```python
from build123d import *

# Parameters (mm, degrees)
BOSS_EXTRUDE1_DEPTH = 50
SKETCH3_W           = 3.3
SKETCH3_H           = 1
BOSS_EXTRUDE2_DEPTH = 13
BOSS_EXTRUDE3_DEPTH = 53.5
CHAMFER1_START      = -14
CHAMFER1_OUTLINE_W  = 52
CHAMFER1_OUTLINE_H  = 13
CHAMFER1_DEPTH      = 3.182909169
CHAMFER2_SIZE       = 3


with BuildPart() as part:
    # Sketch2 → Boss-Extrude1 (new body)
    with BuildSketch(Plane(origin=(0, 0, 0), x_dir=(1, 0, 0), z_dir=(0, 1, 0))):
        Polygon((-1.7, -2), (-1.7, -15), (-5.7, -15), (-5.7, -2), (-9, -2), (-9, -15), (-13, -15), (-13, 2.680601608), align=None)
    extrude(amount=BOSS_EXTRUDE1_DEPTH)

    # Sketch3 → Boss-Extrude2 (add)
    with BuildSketch(Plane.XY.offset(2)):
        with Locations((-7.35, 0.5)):
            Rectangle(SKETCH3_W, SKETCH3_H)
    extrude(amount=BOSS_EXTRUDE2_DEPTH)

    # Sketch5 → Boss-Extrude3 (add)
    with BuildSketch(Plane.XY.offset(15)):
        Polygon((-13, 0), (-1.7, 0), (-1.7, 14), (-5.7, 14), (-5.7, 1), (-9, 1), (-9, 14), (-13, 14), align=None)
    extrude(amount=BOSS_EXTRUDE3_DEPTH)

    # Mirror1: part across plane


with BuildPart() as part_1:
    add(part.part)
    add(part.part.mirror(Plane(origin=(-0.956063716, 0, 2.308147732), x_dir=(0.9238798691632129, 0, 0.38268261961443256), z_dir=(0.3826826196144326, 0, -0.9238798691632131))))

    # Chamfer1: read off the stored shape, not the designer's step
    # Chamfer1 outline → Chamfer1 (cut)
    with BuildSketch(Plane(origin=(0, 0, 0), x_dir=(0, 1, 0), z_dir=(0.9238798691632129, 0, 0.38268261961443295)).offset(CHAMFER1_START)):
        with Locations((25, 2.5)):
            Rectangle(CHAMFER1_OUTLINE_W, CHAMFER1_OUTLINE_H)
    extrude(amount=CHAMFER1_DEPTH, mode=Mode.SUBTRACT)

    # Chamfer2
    chamfer2_edges = [part_1.edges().sort_by_distance(p)[0] for p in [
        (-13, 32, 15),
        (-13, 14, 41.75),
        (-0.497948704, 32, -15.182696898),
        (18.417124413, 14, -34.097836574),
    ]]
    chamfer(chamfer2_edges, length=CHAMFER2_SIZE)


solid = part_1.part
```
Here's how the part is built. I have some questions about the finished solid (model axes, mm). A direction names the side the tool comes from. Give positions to 0.01 mm unless a question says otherwise; leave off trailing zeros. Order: outer loops, then holes, each group sorted by start corner. A loop starts at its lowest first (then second) coordinate and runs counter-clockwise, first axis right, second up. Notation, with made-up numbers: M -28,-2 L 21,-2 A27 ccw 21,23 Z; hole C 61.25,-3.75 d3. An arc over 180 degrees is marked long. Use a Markdown table: item, result. Add a question column.
1. Suppose I cut it at D-D (y = 16). List the corners of the cut face in (x, z) for me.
2. For pin 1 Ø1 at (x, z) = (-7, 46) entering from +Y; pin 2 Ø10 at (y, z) = (15.5, 33.5) entering from +X; pin 3 Ø11.5 at (x, z) = (29.5, -22) entering from +Y; pin 4 Ø10 at (y, z) = (19, 14.5) entering from -X, each with a flat end and sliding along its axis, tell me the tip position at first contact or that it passes through.
3. On a 3-axis mill with a long thin cutter (end or side, diameter ignored), from which of +Z, -Z, +X, -X, +Y, -Y can I reach the whole of each face in a straight line? I mean faces 1 (the flat face through (-11, 13, 40)), 2 (the flat face through (-9, 9, 20)), 3 (the flat face through (-5.7, 25.2, -2)). Say none if no direction works.
4. Suppose I cut it at B-B (z = 37.5). List the corners of the cut face in (x, y) for me.
5. Suppose I cut it at C-C (x = 18). List the corners of the cut face in (y, z) for me.
6. I need wall thicknesses on probe 1 along X at (y, z) = (10.5, 20); probe 2 along X at (y, z) = (11.5, 18); probe 3 along Z at (x, y) = (-6, 6.5). Which ranges of each line are inside material? Lowest first, please. Write a range as from..to.
7. If we mould it in two halves opening along Z, with no side actions, what happens to faces 4 (the flat face through (18, 1, -25)), 5 (the flat face through (25, 14, -27)), 6 (the flat face through (7.26, 10.3, -22.94))? For each: +Z half, -Z half, draft (parallel to the pull), parting line (faces both ways), or undercut.
8. Suppose I cut it at A-A (y = 4). List the corners of the cut face in (x, z) for me, and give its area (4 significant figures).
Results list:
| question | item | result |
|---|---|---|
| 1 | outline | M -13,3.12 L -8.9,-6.78 L -2.62,-13.06 L 1.62,-13.06 L 2.33,-12.35 L -6.86,-3.16 L -4.53,-0.83 L 4.66,-10.02 L 7.49,-7.19 L -1.7,2 L -1.7,15 L -5.7,15 L -5.7,2 L -9,2 L -9,15 L -10,15 L -13,12 Z |
| 2 | pin 1 | stops at y = 1 |
| 2 | pin 2 | stops at x = -1.7 |
| 2 | pin 3 | stops at y = 14 |
| 2 | pin 4 | stops at x = -13 |
| 3 | face 1 | +Z, -X, +Y |
| 3 | face 2 | +Z, +Y |
| 3 | face 3 | +Y |
| 4 | outline | M -13,0 L -1.7,0 L -1.7,14 L -5.7,14 L -5.7,1 L -9,1 L -9,14 L -10,14 L -13,11 Z |
| 5 | outline | M 0,-33.68 L 11,-33.68 L 14,-29.44 L 14,-28.02 L 1,-28.02 L 1,-23.36 L 14,-23.36 L 14,-17.7 L 0,-17.7 Z |
| 6 | probe 1 | x = -13..-9, -5.7..-1.7 |
| 6 | probe 2 | x = -12.5..-9, -5.7..-1.7 |
| 6 | probe 3 | z = -9.68..-4.02, -2.3..2 |
| 7 | face 4 | undercut |
| 7 | face 5 | draft |
| 7 | face 6 | -Z half |
| 8 | outline | M -13,3.12 L -8.9,-6.78 L 37.33,-53.01 L 40.16,-50.18 L -6.86,-3.16 L -4.53,-0.83 L 42.49,-47.85 L 45.32,-45.02 L -1.7,2 L -1.7,68.5 L -5.7,68.5 L -5.7,2 L -9,2 L -9,68.5 L -13,68.5 Z |
| 8 | area | 1,105 mm² |
